from build123d import *

# Parameters (mm, degrees)
SKETCH1_R               = 30.5
BOSS_EXTRUDE1_DEPTH     = 15
SKETCH2_R               = 3.75
BOSS_EXTRUDE2_DEPTH     = 5
CUT_EXTRUDE1_DEPTH      = 49.356100959
CUT_EXTRUDE1_DEPTH_BACK = 49.356100959
SKETCH3_R               = 0.85
CHAMFER1_SIZE           = 1.5
SKETCH4_R               = 7.5
SKETCH4_R_2             = 7
BOSS_EXTRUDE3_DEPTH     = 15


with BuildPart() as part:
    # Sketch1 → Boss-Extrude1 (new body)
    with BuildSketch(Plane.XY):
        Circle(SKETCH1_R)
        with BuildLine():
            ThreePointArc((-25.980383608, -15.000655572), (-28.977676824, -7.764936953), (-30, 0))
            ThreePointArc((-30, 0), (-28.236730197, 10.133462774), (-23.15419548, 19.075723621))
            ThreePointArc((-23.15419548, 19.075723621), (-17.661279409, 0.599319401), (1.158813729, -3.566461936))
            ThreePointArc((1.158813729, -3.566461936), (2.227035272, -3.017086989), (3.06674754, -2.158137977))
            ThreePointArc((3.06674754, -2.158137977), (-7.792065033, -16.868313668), (-25.980383608, -15.000655572))
        make_face(mode=Mode.SUBTRACT)
        with BuildLine():
            ThreePointArc((6.238091175, -29.344270625), (-11.597022419, -27.667834592), (-25.297131148, -16.126225712))
            ThreePointArc((-25.297131148, -16.126225712), (-6.027622102, -16.611674988), (3.75, 0))
            ThreePointArc((3.75, 0), (3.557611987, 1.185705254), (3.000188293, 2.24974892))
            ThreePointArc((3.000188293, 2.24974892), (13.634839116, -12.623289815), (6.238091175, -29.344270625))
        make_face(mode=Mode.SUBTRACT)
        with BuildLine():
            ThreePointArc((29.835735979, -3.135101049), (22.729997369, -19.579254828), (7.519708613, -29.042279221))
            ThreePointArc((7.519708613, -29.042279221), (13.936004079, -10.865899154), (1.158813729, 3.566461936))
            ThreePointArc((1.158813729, 3.566461936), (-0.028310145, 3.749893137), (-1.212529202, 3.548559276))
            ThreePointArc((-1.212529202, 3.548559276), (16.218859038, 9.066691512), (29.835735979, -3.135101049))
        make_face(mode=Mode.SUBTRACT)
        with BuildLine():
            ThreePointArc((1.152171862, 1.25), (0.682388392, -1.557031176), (-1.7, 0))
            ThreePointArc((-1.7, 0), (-1.557031176, 0.682388392), (-1.152171862, 1.25))
            Line((-1.152171862, 1.25), (1.152171862, 1.25))
        make_face(mode=Mode.SUBTRACT)
        with BuildLine():
            ThreePointArc((-1.104834079, -3.583551543), (-18.450600149, 2.198098635), (-22.294851286, 20.073355628))
            ThreePointArc((-22.294851286, 20.073355628), (-6.880556914, 29.200307131), (10.987051359, 27.91567127))
            ThreePointArc((10.987051359, 27.91567127), (-4.887648858, 16.982074748), (-3.033813729, -2.204194696))
            ThreePointArc((-3.033813729, -2.204194696), (-2.181228495, -3.05036756), (-1.104834079, -3.583551543))
        make_face(mode=Mode.SUBTRACT)
        with BuildLine():
            ThreePointArc((-3.033813729, 2.204194696), (-3.566461936, 1.158813729), (-3.75, 0))
            ThreePointArc((-3.75, 0), (-3.749893137, -0.028310145), (-3.749572552, -0.056618677))
            ThreePointArc((-3.749572552, -0.056618677), (-3.611032972, 18.226813335), (12.201407739, 27.406671618))
            ThreePointArc((12.201407739, 27.406671618), (25.644933357, 15.567189634), (29.944566656, -1.822889958))
            ThreePointArc((29.944566656, -1.822889958), (14.64054629, 9.896179992), (-3.033813729, 2.204194696))
        make_face(mode=Mode.SUBTRACT)
    extrude(amount=BOSS_EXTRUDE1_DEPTH)

    # Sketch2 → Boss-Extrude2 (add)
    with BuildSketch(Plane.XY.offset(15)):
        Circle(SKETCH2_R)
        with BuildLine():
            Line((-1.152171862, 1.25), (1.152171862, 1.25))
            ThreePointArc((1.152171862, 1.25), (0, -1.7), (-1.152171862, 1.25))
        make_face(mode=Mode.SUBTRACT)
    extrude(amount=BOSS_EXTRUDE2_DEPTH)

    # Sketch3 → Cut-Extrude1 (cut, two sides: drawn at the far end of the back side and taken through both)
    with BuildSketch(Plane.XZ.offset(-1.25).offset(-CUT_EXTRUDE1_DEPTH_BACK)):
        with Locations(Location((0, 17.5, 0), (0, 0, 270))):
            Circle(SKETCH3_R)
    extrude(amount=CUT_EXTRUDE1_DEPTH + CUT_EXTRUDE1_DEPTH_BACK, mode=Mode.SUBTRACT)

    # Chamfer1
    chamfer1_edges = [part.edges().sort_by_distance(p)[0] for p in [
        (-3.75, 0, 20),
    ]]
    chamfer(chamfer1_edges, length=CHAMFER1_SIZE)

    # Sketch4 → Boss-Extrude3 (add)
    with BuildSketch(Plane(origin=(0, 0, 0), x_dir=(-1, 0, 0), z_dir=(0, 0, -1))):
        Circle(SKETCH4_R)
        Circle(SKETCH4_R_2, mode=Mode.SUBTRACT)
    extrude(amount=-BOSS_EXTRUDE3_DEPTH)


solid = part.part
Model file for the job. Use its own axes, mm. Coordinates: 2 decimals unless noted, no trailing zeros. Loops run counter-clockwise (first coordinate to the right, second up) from the corner with the lowest first, then second, coordinate; pieces in that order, holes last. Notation, with made-up numbers: (49, -37) -> (98, -37) arc R31 ccw to (98, -4) -> close; hole circle Ø8 at (-12, 23.25). An arc over 180 degrees is marked (long way). Use one line per item in the form item = value. Start each with the question number.
(1) Cut at C-C on x = 23.5. Give the cut face in (y, z).
(2) Probe probe 1 along X at (y, z) = (15, 5); probe 2 along X at (y, z) = (-10.5, 10); probe 3 along X at (y, z) = (-25.5, 9). List the from-to ranges inside material, lowest first. Write a range as from..to.
(3) Cut at A-A on z = 17.5. Give the cut face in (x, y).
(4) Cut at B-B on y = -26. Give the cut face in (x, z).
(5) Cut at D-D on y = 11.5. Give the cut face in (x, z), and give its area (3 significant figures).
(6) Flat gauge pins, fed straight in: pin 1 (2.5 mm diameter, centred on x = 0, z = 17.5, fed in from -Y); pin 2 (12 mm diameter, centred on x = -20.5, z = 10.5, fed in from +Y); pin 3 (1 mm diameter, centred on y = 14, z = 10.5, fed in from -X). Where does each tip first touch, or does it go through?
(7) Pull direction X, two halves, no side cores. Call faces 1 (the cylindrical face through (-4.758, 2.043, 7.395)), 2 (the flat face through (2, 0, 0)): pulls with the +X half, pulls with the -X half, needs draft (parallel to the pull), parting line crosses it, or undercut.
Values:
q1.outline = (-19.44, 0) -> (-18.65, 0) -> (-18.65, 15) -> (-19.44, 15) -> close; (5.72, 0) -> (6.41, 0) -> (6.41, 15) -> (5.72, 15) -> close; (18.65, 0) -> (19.44, 0) -> (19.44, 15) -> (18.65, 15) -> close
q2.probe_1 = -26.56..-25.98, -23.71..-23.15, -5.68..-5.09, 25.98..26.56
q2.probe_2 = -28.64..-28.1, -0.09..0.59, 13.29..13.86, 28.1..28.64
q2.probe_3 = -16.73..-15.8, 10.09..10.78, 15.8..16.73
q3.outline = (-1.15, 1.25) -> (-0.85, 1.25) -> (-0.85, 3.65) arc R3.75 ccw to (-0.85, -3.65) -> (-0.85, -1.47) arc R1.7 cw to start; (0.85, -3.65) arc R3.75 ccw to (0.85, 3.65) -> (0.85, 1.25) -> (1.15, 1.25) arc R1.7 cw to (0.85, -1.47) -> close
q4.outline = (-15.95, 0) -> (-14.97, 0) -> (-14.97, 15) -> (-15.95, 15) -> close; (9.71, 0) -> (10.41, 0) -> (10.41, 15) -> (9.71, 15) -> close; (14.97, 0) -> (15.95, 0) -> (15.95, 15) -> (14.97, 15) -> close
q5.outline = (-28.25, 0) -> (-27.71, 0) -> (-27.71, 15) -> (-28.25, 15) -> close; (-23.47, 0) -> (-22.91, 0) -> (-22.91, 15) -> (-23.47, 15) -> close; (-6.49, 0) -> (-5.93, 0) -> (-5.93, 15) -> (-6.49, 15) -> close; (27.71, 0) -> (28.25, 0) -> (28.25, 15) -> (27.71, 15) -> close
q5.area = 33.1 mm2
q6.pin_1 = -3.75
q6.pin_2 = 26.83
q6.pin_3 = -27.35
q7.face_1 = undercut
q7.face_2 = needs draft
